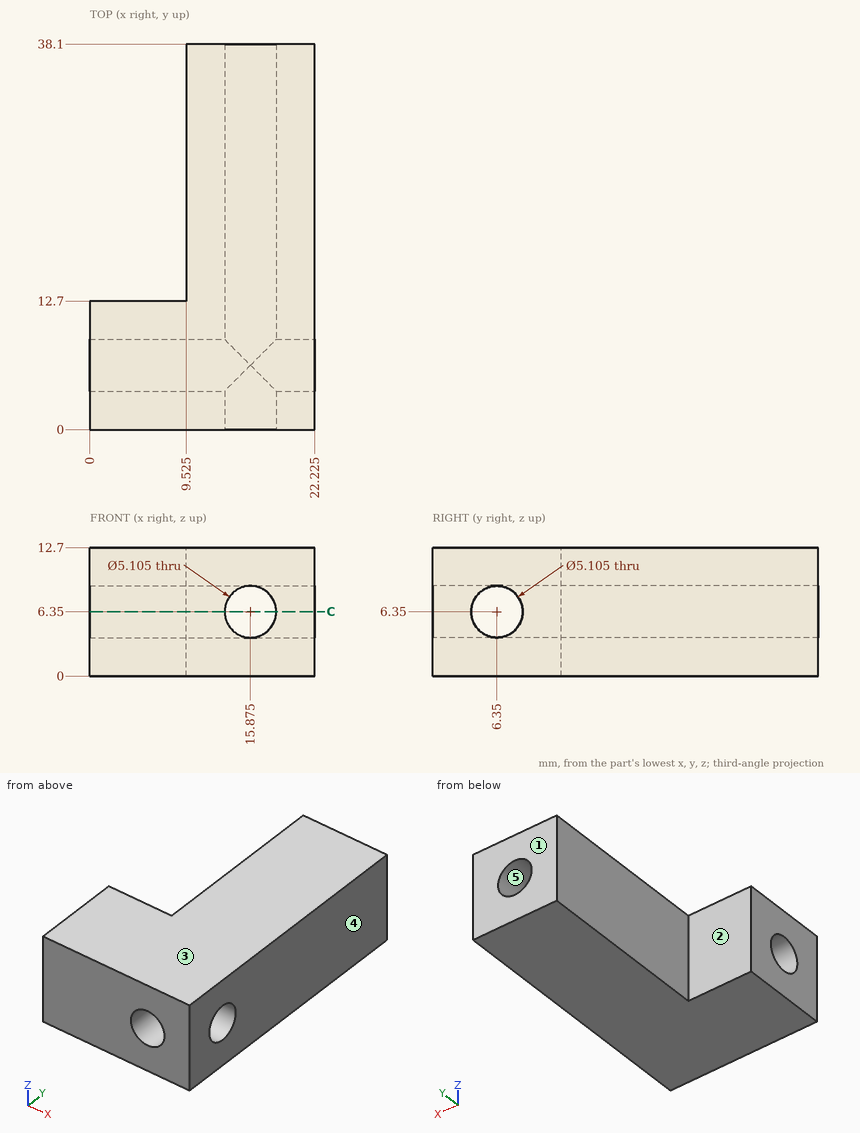
Geometry: see drawing. Coordinates: mm, zero at the bounding-box minimum. A direction names the side the tool comes from. Give positions to 0.01 mm unless a question says otherwise; leave off trailing zeros. Loops run counter-clockwise (first coordinate to the right, second up) from the corner with the lowest first, then second, coordinate; pieces in that order, holes last. Notation, with made-up numbers: (-30.75, 42.5) - (-17.75, 42.5) arc R23 ccw to (-17.75, 62.5) - close; hole circle Ø9 at (13.25, 82). An arc over 180 degrees is marked (long way). Use CSV: the item, a comma, the result in double quotes. Start each with the question number.
1. Pin query (flat end, axial travel): pin 1 (5 mm diameter, centred on x = 3.5, z = 5.5, fed in from +Y); pin 2 (1.5 mm diameter, centred on y = 30.5, z = 8, fed in from -X) (3 decimals). Return the tip coordinate at first contact, or that it passes through.
2. Section C-C (z = 6.35). Output: boundary loops of the cut face in (x, y) (1 decimal), then the cut area to 3 significant figures.
3. Ray query, L1, parallel to Z at x = 20.5, y = 6.35; L2, parallel to Y at x = 19, z = 6.35. Return the intervals inside material, ascending.
4. Reachability of the marked faces 1 and 2 from +Z, -Z, +X, -X, +Y, -Y: full face, straight path, thin tool, end or side. Return the list, or none.
5. Draft query along Z for the marked faces 3, 4 and 5. Return one class per face: +Z half, -Z half, draft (parallel to the pull), parting line (faces both ways), or undercut.
Response:
1,pin 1,"y = 12.7"
1,pin 2,"x = 9.525"
2,outline,"(0, 0) - (13.3, 0) - (13.3, 3.8) - (0, 3.8) - close; (0, 8.9) - (13.3, 8.9) - (13.3, 38.1) - (9.5, 38.1) - (9.5, 12.7) - (0, 12.7) - close; (18.4, 0) - (22.2, 0) - (22.2, 3.8) - (18.4, 3.8) - close; (18.4, 8.9) - (22.2, 8.9) - (22.2, 38.1) - (18.4, 38.1) - close"
2,area,"323 mm²"
3,L1,"0 to 3.8, 8.9 to 12.7"
3,L2,"0 to 3.8, 8.9 to 38.1"
4,face 1,"+Z, -Z, +X, -X, +Y"
4,face 2,"+Z, -Z, -X, +Y"
5,face 3,"+Z half"
5,face 4,"draft"
5,face 5,"undercut"
